Part model, mm, in its own coordinate system. A direction names the side the tool comes from. Round coordinates to 2 decimals unless told otherwise and drop trailing zeros. Order: outer loops, then holes, each group sorted by start corner. A loop starts at its lowest first (then second) coordinate and runs counter-clockwise, first axis right, second up. Notation, with made-up numbers: M -14,-21.75 L 4,-21.75 A18 cw 4,0.25 Z; hole C -34.5,-35 d5. An arc over 180 degrees is marked long. Write each question's results on one line, items separated by ' | '. Start each with the question number.
1. Band-saw the part on D-D, the plane x = -7.25. List the corners of the cut face in (y, z).
2. Band-saw the part on B-B, the plane y = 1.75. List the corners of the cut face in (x, z), then the cut area to 3 significant figures.
3. Band-saw the part on A-A, the plane z = 1.5. List the corners of the cut face in (x, y) (3 decimals), then the cut area to 3 significant figures.
4. Band-saw the part on C-C, the plane z = 9.5. List the corners of the cut face in (x, y), then the cut area to 3 significant figures.
5. Two-plate mould, pull along Y, no slides. Class faces 1 (the face through (-2, 2, 4.805)), 2 (the face through (-7, 1, 5)), 3 (the face through (-2.5, 3.2, 9.21)): +Y half, -Y half, draft (parallel to the pull), parting line (faces both ways), or undercut.
6. Drop flat-ended pins along their axis: pin 1 Ø1.2 at (x, z) = (-2.5, 2.5) entering from -Y; pin 2 Ø0.8 at (x, y) = (-7.5, 3.5) entering from +Z. Give the stop position or say it passes through.
7. Which spindle directions (+Z, -Z, +X, -X, +Y, -Y) get a long thin tool onto all of the face, cutting with end or side? Do faces 4 (the face through (-1.5, 3.2, 9.71)), 5 (the face through (-9.025, 2, 4)), 6 (the face through (-5, 0, 3)). Say none if no direction does.
8. Probe L1, parallel to X at y = 4.5, z = 9.25; L2, parallel to X at y = 1.25, z = 3.25; L3, parallel to Z at x = -8, y = 2. List the from-to ranges inside material, lowest first. Write a range as [from, to].
```python
from build123d import *

# Parameters (mm, degrees)
CROQUIS1_W              = 9.95
CROQUIS1_H              = 7.49
SALIENTE_EXTRUIR1_DEPTH = 10.21
CORTAR_EXTRUIR1_DEPTH   = 17.104244782
CROQUIS3_W              = 3.98
CROQUIS3_H              = 5.08
CORTAR_EXTRUIR3_DEPTH   = 1
CROQUIS4_R              = 1.69
CORTAR_EXTRUIR4_DEPTH   = 0.5
CORTAR_EXTRUIR6_DEPTH   = 0.5
CROQUIS7_W              = 3.119915204
CROQUIS7_H              = 2.530639344
CORTAR_EXTRUIR7_DEPTH   = 2


with BuildPart() as part:
    # Croquis1 → Saliente-Extruir1 (new body)
    with BuildSketch(Plane.XY):
        with Locations((-4.975, 3.745)):
            Rectangle(CROQUIS1_W, CROQUIS1_H)
    extrude(amount=SALIENTE_EXTRUIR1_DEPTH)

    # Croquis2 → Cortar-Extruir1 (cut, through all)
    with BuildSketch(Plane.ZY.offset(9.95)):
        Polygon((10.21, 5.699503954), (10.21, 7.49), (6.5, 7.49), align=None)
        Polygon((10.21, 0.7), (10.21, 0), (6.5, 0), align=None)
    extrude(amount=-CORTAR_EXTRUIR1_DEPTH, mode=Mode.SUBTRACT)

    # Croquis3 → Cortar-Extruir3 (cut)
    with BuildSketch(Plane(origin=(0, 0, 0), x_dir=(-1, 0, 0), z_dir=(0, -1, 0))):
        with Locations((2.485, -3.54)):
            Rectangle(CROQUIS3_W, CROQUIS3_H)
        with Locations((7.465, -3.54)):
            Rectangle(CROQUIS3_W, CROQUIS3_H)
    extrude(amount=-CORTAR_EXTRUIR3_DEPTH, mode=Mode.SUBTRACT)

    # Croquis4 → Cortar-Extruir4 (cut)
    with BuildSketch(Plane.XY.offset(10.21)):
        with Locations((-2.4875, 3.199751977)):
            Circle(CROQUIS4_R)
        with Locations(Location((-7.4625, 3.199751977, 0), (0, 0, 180))):
            Circle(CROQUIS4_R)
    extrude(amount=-CORTAR_EXTRUIR4_DEPTH, mode=Mode.SUBTRACT)

    # Croquis6 → Cortar-Extruir6 (cut)
    with BuildSketch(Plane.XY.offset(9.71)):
        with BuildLine():
            Line((-6.96704565, 1.584009118), (-6.96704565, 4.815494836))
            ThreePointArc((-6.96704565, 4.815494836), (-7.4625, 4.889751977), (-7.95795435, 4.815494836))
            Line((-7.95795435, 4.815494836), (-7.95795435, 1.584009118))
            ThreePointArc((-7.95795435, 1.584009118), (-7.4625, 1.509751977), (-6.96704565, 1.584009118))
        make_face()
        with BuildLine():
            Line((-1.99204565, 1.584009118), (-1.99204565, 4.815494836))
            ThreePointArc((-1.99204565, 4.815494836), (-2.4875, 4.889751977), (-2.98295435, 4.815494836))
            Line((-2.98295435, 4.815494836), (-2.98295435, 1.584009118))
            ThreePointArc((-2.98295435, 1.584009118), (-2.4875, 1.509751977), (-1.99204565, 1.584009118))
        make_face()
    extrude(amount=-CORTAR_EXTRUIR6_DEPTH, mode=Mode.SUBTRACT)

    # Croquis7 → Cortar-Extruir7 (cut)
    with BuildSketch(Plane(origin=(0, 1, 0), x_dir=(-1, 0, 0), z_dir=(0, -1, 0))):
        with Locations((7.465, -3.54)):
            Rectangle(CROQUIS7_W, CROQUIS7_H)
        with Locations((2.485, -3.54)):
            Rectangle(CROQUIS7_W, CROQUIS7_H)
    extrude(amount=-CORTAR_EXTRUIR7_DEPTH, mode=Mode.SUBTRACT)


solid = part.part
```
Solution:
1) outline: M 0,0 L 7.49,0 L 7.49,6.5 L 5.7,10.21 L 4.88,10.21 L 4.88,9.21 L 1.52,9.21 L 1.52,10.21 L 0.7,10.21 L 0,6.5 L 0,6.08 L 1,6.08 L 1,4.81 L 3,4.81 L 3,2.27 L 1,2.27 L 1,1 L 0,1 Z
2) outline: M -9.95,0 L 0,0 L 0,10.21 L -1.62,10.21 L -1.62,9.71 L -1.99,9.71 L -1.99,9.21 L -2.98,9.21 L -2.98,9.71 L -3.36,9.71 L -3.36,10.21 L -6.59,10.21 L -6.59,9.71 L -6.97,9.71 L -6.97,9.21 L -7.96,9.21 L -7.96,9.71 L -8.33,9.71 L -8.33,10.21 L -9.95,10.21 Z; hole M -9.02,2.27 L -5.91,2.27 L -5.91,4.81 L -9.02,4.81 Z; hole M -4.04,2.27 L -0.93,2.27 L -0.93,4.81 L -4.04,4.81 Z | area: 83.1 mm^2
3) outline: M -9.95,0 L -9.455,0 L -9.455,1 L -5.475,1 L -5.475,0 L -4.475,0 L -4.475,1 L -0.495,1 L -0.495,0 L 0,0 L 0,7.49 L -9.95,7.49 Z | area: 66.6 mm^2
4) outline: M -9.95,0.57 L 0,0.57 L 0,6.04 L -9.95,6.04 Z; hole M -7.96,1.58 A1.69 ccw -6.97,1.58 L -6.97,4.82 A1.69 ccw -7.96,4.82 Z; hole M -2.98,1.58 A1.69 ccw -1.99,1.58 L -1.99,4.82 A1.69 ccw -2.98,4.82 Z | area: 47.9 mm^2
5) face 1: draft | face 2: -Y half | face 3: undercut
6) pin 1: y = 1 | pin 2: z = 9.21
7) face 4: +Z | face 5: -Y | face 6: +Z, -Z, +X, -X, -Y
8) L1: [-9.95, -7.96], [-6.97, -2.98], [-1.99, 0] | L2: [-9.95, -9.02], [-5.91, -4.04], [-0.93, 0] | L3: [0, 2.27], [4.81, 9.71]
